Print and shaded views of the part. All mm, measured from the part's lowest x, y and z. A direction names the side the tool comes from. Round coordinates to 2 decimals unless told otherwise and drop trailing zeros. Write each loop counter-clockwise with the first axis right and the second up, starting at its lowest first coordinate (ties: lowest second). Pieces come first, ordered by that corner, then holes. Notation, with made-up numbers: (36.5, 57) - (82.5, 57) arc R6 cw to (82.5, 67) - close; hole circle Ø3 at (10.5, 88.5). An arc over 180 degrees is marked (long way). Answer as a JSON object with one key per item and string values. Group by question number.
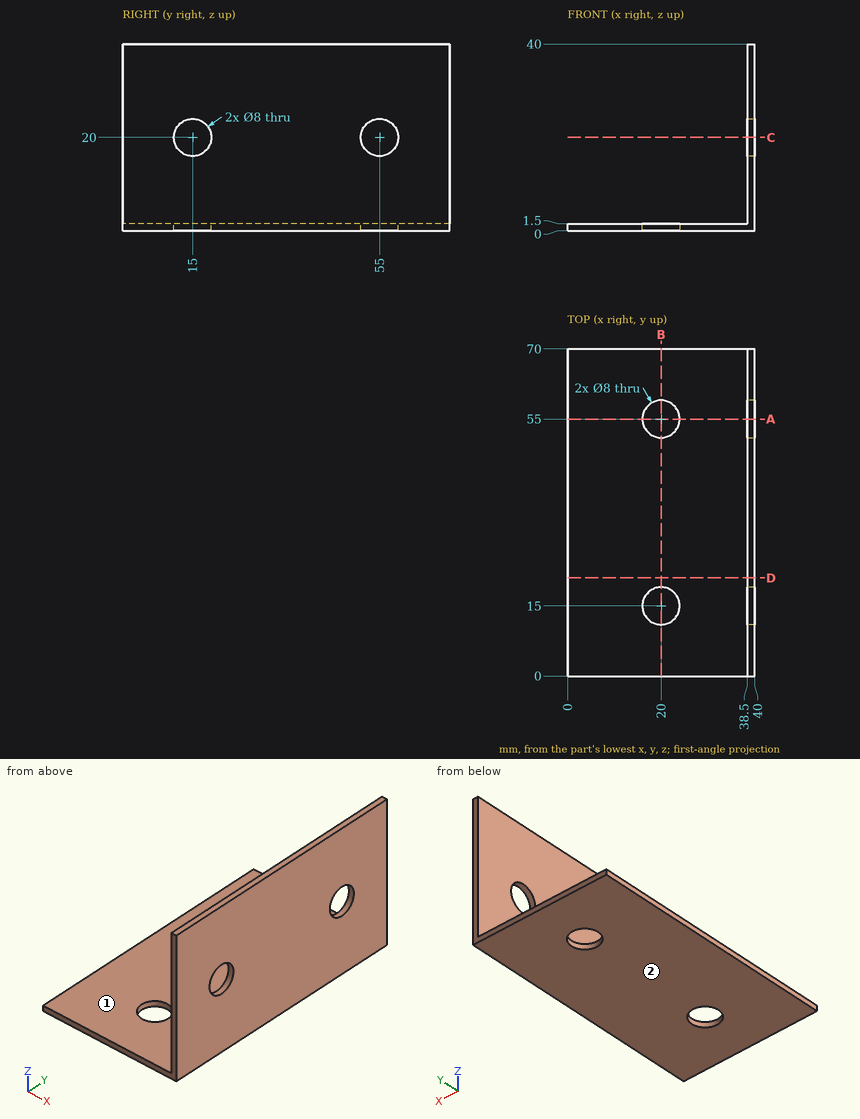
(1) Slice it at C-C (z = 20). Write the cut outline in (x, y), then the cut area to 3 significant figures.
(2) Slice it at D-D (y = 21). Write the cut outline in (x, z), then the cut area to 3 significant figures.
(3) Slice it at A-A (y = 55). Write the cut outline in (x, z), then the cut area to 4 significant figures.
(4) Drill centre lines: line 1 (Y direction, x = 20, z = 0.55); line 2 (X direction, y = 50, z = 12.5); line 3 (Z direction, x = 12.5, y = 5). Where is each one in solid material? Low to high. Write a range as from..to.
(5) 3-axis set-ups, long thin cutter, end or side, ignore diameter. For the marked faces 1 and 2: which of +Z, -Z, +X, -X, +Y, -Y reach the whole face in a straight line?
(6) Slice it at B-B (x = 20). Write the cut outline in (y, z), then the cut area to 3 significant figures.
(7) Flat gauge pins, fed straight in: pin 1 (10.5 mm diameter, centred on x = 20, y = 55, fed in from +Z); pin 2 (4 mm diameter, centred on y = 32, z = 27.5, fed in from -X). Where does each tip first touch, or does it go through?
Answer:
{
 "1": {"outline": "(38.5, 0) - (40, 0) - (40, 11) - (38.5, 11) - close; (38.5, 19) - (40, 19) - (40, 51) - (38.5, 51) - close; (38.5, 59) - (40, 59) - (40, 70) - (38.5, 70) - close", "area": "81.0 mm²"},
 "2": {"outline": "(0, 0) - (40, 0) - (40, 40) - (38.5, 40) - (38.5, 1.5) - (0, 1.5) - close", "area": "118 mm²"},
 "3": {"outline": "(0, 0) - (16, 0) - (16, 1.5) - (0, 1.5) - close; (24, 0) - (40, 0) - (40, 16) - (38.5, 16) - (38.5, 1.5) - (24, 1.5) - close; (38.5, 24) - (40, 24) - (40, 40) - (38.5, 40) - close", "area": "93.75 mm²"},
 "4": {"line 1": "0..11, 19..51, 59..70", "line 2": "38.5..40", "line 3": "0..1.5"},
 "5": {"face 1": "+Z, -X, +Y, -Y", "face 2": "-Z, +X, -X, +Y, -Y"},
 "6": {"outline": "(0, 0) - (11, 0) - (11, 1.5) - (0, 1.5) - close; (19, 0) - (51, 0) - (51, 1.5) - (19, 1.5) - close; (59, 0) - (70, 0) - (70, 1.5) - (59, 1.5) - close", "area": "81.0 mm²"},
 "7": {"pin 1": "z = 1.5", "pin 2": "x = 38.5"}
}
